Autodesk Inventor part; units mm, degrees
ref_plane "YZ Plane" through (0, 0, 0) normal (1, 0, 0) x (0, 1, 0)
ref_plane "XZ Plane" through (0, 0, 0) normal (0, 1, 0) x (-1, 0, 0)
ref_plane "XY Plane" through (0, 0, 0) normal (0, 0, 1) x (1, 0, 0)
sketch "スケッチ1" plane through (0, 0, 0) normal (0, 0, 1) x (1, 0, 0)
  line L0 (-28, -52.5) -> (28, -52.5) construction
  line L1 (28, -52.5) -> (28, 52.5) construction
  line L2 (28, 52.5) -> (-28, 52.5) construction
  line L3 (-28, 52.5) -> (-28, -52.5) construction
  line L4 (-28, -52.5) -> (28, 52.5) construction
  line L5 (28, -52.5) -> (-28, 52.5) construction
  line L6 (-28, -52.5) -> (-28, 52.5)
  line L7 (-28, 52.5) -> (28, 52.5)
  line L8 (28, 52.5) -> (28, -52.5)
  line L9 (-28, -52.5) -> (28, -52.5)
  line L10 (0, 0) -> (0, 52.5) construction
  line L11 (0, 0) -> (28, 0) construction
  line L12 (-24.5, 44.5) -> (24.5, 44.5) construction
  line L13 (24.5, 44.5) -> (24.5, -13.5) construction
  line L14 (24.5, -13.5) -> (-24.5, -13.5) construction
  line L15 (-24.5, -13.5) -> (-24.5, 44.5) construction
  line L16 (-24.5, 44.5) -> (24.5, -13.5) construction
  line L17 (24.5, 44.5) -> (-24.5, -13.5) construction
  circle A0 centre (-24.5, 44.5) radius 1.04
  circle A1 centre (-24.5, -13.5) radius 1.04
  circle A2 centre (24.5, -13.5) radius 1.04
  circle A3 centre (24.5, 44.5) radius 1.04
  point P0 (0, 15.5)
  point P1 (0, 15.5)
  point P2 (0, 0)
  dimension "d9" = 56
  dimension "d12" = 105
  dimension "d52" = 2.08
  dimension "d53" = 49
  dimension "d54" = 58
  dimension "d55" = 8
extrude "押し出し1" add sketch "スケッチ1" along normal blind 5
sketch "スケッチ3" plane through (0, 0, 5) normal (0, 0, 1) x (1, 0, 0)
  line L0 (28, 52.5) -> (-28, 52.5)
  line L1 (-28, 52.5) -> (-28, -52.5)
  line L2 (-20, -44.5) -> (20, -44.5)
  line L3 (20, -44.5) -> (20, 44.5)
  line L4 (20, 44.5) -> (-20, 44.5)
  line L5 (-20, 44.5) -> (-20, -44.5)
  line L6 (-20, -44.5) -> (20, 44.5) construction
  line L7 (20, -44.5) -> (-20, 44.5) construction
  point P0 (-28, 42.1)
  point P1 (0, 0)
  dimension "d47" = 8
  dimension "d48" = 8
extrude "押し出し3" cut sketch "スケッチ3" against normal blind 10
fillet "フィレット1" radius 10 4 edges at (-20, 44.5, 2.5) (20, 44.5, 2.5) (20, -44.5, 2.5) (-20, -44.5, 2.5)
sketch "スケッチ4" plane through (-28, -52.5, 0) normal (-1, 0, 0) x (0, 0, 1)
  line L0 (0, 0) -> (5, 0)
  line L1 (0, 105) -> (5, 105)
  point P0 (0, 52.5)
  point P1 (2.5, 90)
  point P2 (2.5, 15)
  point P3 (2.5, 105)
  dimension "d73" = 15
  dimension "d74" = 15
hole "穴1" at (-28, 37.5, 2.5) at (-28, -37.5, 2.5) direction (1, 0, 0) diameter 2.459 depth 2.5
mirror "ミラー1" about plane through (0, 0, 0) normal (1, 0, 0) of "穴1"
equation "\"d12\" = d19"
equation "\"d55\" = d69"
equation "\"d47\" = d48"
properties part number "コックピット_2_サブフレーム_1" material "アセタール樹脂、黒"
The listing builds one solid part. Answer for the finished solid, in the listing's coordinates (mm). A direction names the side the tool comes from. Give positions to 0.01 mm unless a question says otherwise; leave off trailing zeros. Order: outer loops, then holes, each group sorted by start corner. A loop starts at its lowest first (then second) coordinate and runs counter-clockwise, first axis right, second up.
Item 1: Given pin 1 Ø1.2 at (x, y) = (24.5, -13.5) entering from -Z; pin 2 Ø1.2 at (y, z) = (37.5, 2.5) entering from -X, each flat-ended and moving along its own axis, determine where each tip first touches the part or whether it passes through.
From the geometry:
pin 1: passes through
pin 2: stops at x = -25.5
Item 2: The part is cut by section A-A, the plane x = 24.5. Give the vertices of the cut face in (y, z), and give its area (3 significant figures).
From the geometry:
outline: (-52.5, 0) - (-14.54, 0) - (-14.54, 5) - (-52.5, 5) - close; (-12.46, 0) - (43.46, 0) - (43.46, 5) - (-12.46, 5) - close; (45.54, 0) - (52.5, 0) - (52.5, 5) - (45.54, 5) - close
area: 504 mm2
Item 3: The part is cut by section D-D, the plane y = 14.5. Give the vertices of the cut face in (x, z), and give its area (3 significant figures).
From the geometry:
outline: (-28, 0) - (-20, 0) - (-20, 5) - (-28, 5) - close; (20, 0) - (28, 0) - (28, 5) - (20, 5) - close
area: 80.0 mm2
Item 4: The part is cut by section C-C, the plane z = 2.5. Count the separate pieces of the cut face and the enclosed holes in it, and give its area (3 significant figures).
From the geometry:
separate pieces: 1
enclosed holes: 5
area: 2,370 mm2
Item 5: For a pull along Y with two mould halves and no side action, classify faces 1 (the face through (0, -52.5, 2)), 2 (the face through (-25, 1, 5)), 3 (the face through (25.5, -38, 3)), 4 (the face through (17.15, -41.49, 2.46)) as pulls with the +Y half, pulls with the -Y half, needs draft (parallel to the pull), parting line crosses it, or undercut.
From the geometry:
face 1: pulls with the -Y half
face 2: needs draft
face 3: undercut
face 4: undercut
Item 6: The part is cut by section B-B, the plane y = -13.5. Give the vertices of the cut face in (x, z).
From the geometry:
outline: (-28, 0) - (-25.54, 0) - (-25.54, 5) - (-28, 5) - close; (-23.46, 0) - (-20, 0) - (-20, 5) - (-23.46, 5) - close; (20, 0) - (23.46, 0) - (23.46, 5) - (20, 5) - close; (25.54, 0) - (28, 0) - (28, 5) - (25.54, 5) - close
Item 7: Find the intervals of material crossed by probe 1 along Y at (x, z) = (24.5, 1); probe 2 along Y at (x, z) = (27.1, 2.5); probe 3 along Y at (x, z) = (-6, 2.25), in increasing order.
From the geometry:
probe 1: y = -52.5 to -14.54, -12.46 to 43.46, 45.54 to 52.5
probe 2: y = -52.5 to -38.73, -36.27 to 36.27, 38.73 to 52.5
probe 3: y = -52.5 to -44.5, 44.5 to 52.5
Item 8: Which of the six approach directions +Z, -Z, +X, -X, +Y, -Y give full straight-line access (tool end or side, diameter ignored) to faces 5 (the face through (26.73, 38.72, 2.34)), 6 (the face through (0, 44.5, 3)), 7 (the face through (-25.5, -38, 2))?
From the geometry:
face 5: +X
face 6: +Z, -Z
face 7: -X
